Input: part model. Units: mm. Frame: model coordinates. Give positions to 0.01 mm unless a question says otherwise; leave off trailing zeros. Write each loop counter-clockwise with the first axis right and the second up, starting at its lowest first coordinate (ties: lowest second). Pieces come first, ordered by that corner, then holes.
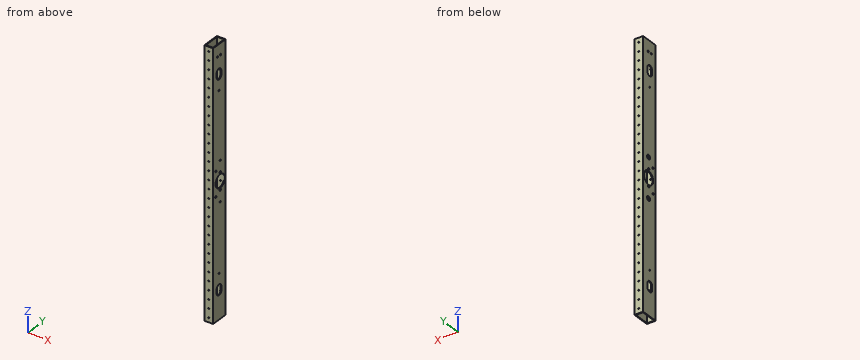
```python
from build123d import *

# Parameters (mm, degrees)
SKETCH1_W           = 25.4
SKETCH1_H           = 50.8
SKETCH1_W_2         = 20.32
SKETCH1_H_2         = 45.72
EXTRUDE_THIN1_DEPTH = 381
SKETCH3_R           = 1.5875
CUT_EXTRUDE2_DEPTH  = 51.8
LPATTERN1_COUNT     = 220
LPATTERN1_PITCH     = 25.4
SKETCH6_R           = 19.05
SKETCH6_R_2         = 3.175
CUT_EXTRUDE5_DEPTH  = 26.4
SKETCH4_R           = 9.525
CUT_EXTRUDE3_DEPTH  = 26.4
CUT_EXTRUDE6_START  = -22.86
SKETCH7_R           = 6.35
CUT_EXTRUDE6_DEPTH  = 2.54
SKETCH8_R           = 2.5273
CUT_EXTRUDE7_DEPTH  = 26.4
SKETCH9_R           = 2.0193
CUT_EXTRUDE8_DEPTH  = 26.4
SKETCH10_R          = 2.4892
CUT_EXTRUDE9_DEPTH  = 26.4
SKETCH11_R          = 2.413
CUT_EXTRUDE10_DEPTH = 26.4


with BuildPart() as part:
    # Sketch1 → Extrude-Thin1 (new body, symmetric)
    with BuildSketch(Plane.XY):
        with Locations((12.7, 25.4)):
            Rectangle(SKETCH1_W, SKETCH1_H)
        with Locations((12.7, 25.4)):
            Rectangle(SKETCH1_W_2, SKETCH1_H_2, mode=Mode.SUBTRACT)
    extrude(amount=EXTRUDE_THIN1_DEPTH, both=True)

    # Sketch3 → Cut-Extrude2 (cut, through all)
    with BuildSketch(Plane(origin=(0, 50.8, 0), x_dir=(1, 0, 0), z_dir=(0, 1, 0))):
        with Locations((12.7, -368.3)):
            Circle(SKETCH3_R)
    cut_extrude2 = extrude(amount=-CUT_EXTRUDE2_DEPTH, mode=Mode.SUBTRACT)

    # LPattern1: Cut-Extrude2 ×220
    with Locations(*[(0, 0, -i * LPATTERN1_PITCH) for i in range(1, LPATTERN1_COUNT)]):
        add(cut_extrude2, mode=Mode.SUBTRACT)

    # Sketch6 → Cut-Extrude5 (cut, through all)
    with BuildSketch(Plane(origin=(25.4, 0, 0), x_dir=(0, 0, -1), z_dir=(1, 0, 0))):
        with Locations((0, 28.7655)):
            Circle(SKETCH6_R)
        with Locations((23.8125, 28.7655)):
            Circle(SKETCH6_R_2)
        with Locations((-23.8125, 28.7655)):
            Circle(SKETCH6_R_2)
    extrude(amount=-CUT_EXTRUDE5_DEPTH, mode=Mode.SUBTRACT)

    # Sketch4 → Cut-Extrude3 (cut, through all)
    with BuildSketch(Plane(origin=(25.4, 0, 0), x_dir=(0, 0, -1), z_dir=(1, 0, 0))):
        with Locations((295.234514267, 23.876)):
            Circle(SKETCH4_R)
        with BuildLine():
            Line((304.124514267, 33.401), (295.234514267, 33.401))
            ThreePointArc((295.234514267, 33.401), (301.969706358, 30.611192091), (304.759514267, 23.876))
            ThreePointArc((304.759514267, 23.876), (301.969706356, 17.140807907), (295.234514261, 14.351))
            Line((295.234514261, 14.351), (304.124514267, 14.351))
            ThreePointArc((304.124514267, 14.351), (313.649514267, 23.876), (304.124514267, 33.401))
        make_face()
        with BuildLine():
            Line((295.234514267, 33.401), (292.694514267, 33.401))
            ThreePointArc((292.694514267, 33.401), (283.169514267, 23.876), (292.694514267, 14.351))
            Line((292.694514267, 14.351), (295.234514261, 14.351))
            ThreePointArc((295.234514261, 14.351), (285.709514267, 23.876000003), (295.234514267, 33.401))
        make_face()
    cut_extrude3 = extrude(amount=-CUT_EXTRUDE3_DEPTH, mode=Mode.SUBTRACT)

    # Mirror1: Cut-Extrude3 across plane
    add(cut_extrude3.mirror(Plane.XY), mode=Mode.SUBTRACT)

    # Sketch7 → Cut-Extrude6 (cut)
    with BuildSketch(Plane(origin=(25.4, 0, 0), x_dir=(0, 0, -1), z_dir=(1, 0, 0)).offset(CUT_EXTRUDE6_START)):
        with Locations((57.15, 28.7655)):
            Circle(SKETCH7_R)
        with Locations((-57.15, 28.7655)):
            Circle(SKETCH7_R)
    extrude(amount=-CUT_EXTRUDE6_DEPTH, mode=Mode.SUBTRACT)

    # Sketch8 → Cut-Extrude7 (cut, through all)
    with BuildSketch(Plane(origin=(25.4, 0, 0), x_dir=(0, 0, -1), z_dir=(1, 0, 0))):
        with Locations((-35.41150672, 10.9347)):
            Circle(SKETCH8_R)
        with Locations((35.41150672, 10.9347)):
            Circle(SKETCH8_R)
    extrude(amount=-CUT_EXTRUDE7_DEPTH, mode=Mode.SUBTRACT)

    # Sketch9 → Cut-Extrude8 (cut, through all)
    with BuildSketch(Plane.ZY):
        with Locations((252.689514267, 23.876)):
            Circle(SKETCH9_R)
    cut_extrude8 = extrude(amount=-CUT_EXTRUDE8_DEPTH, mode=Mode.SUBTRACT)

    # Mirror2: Cut-Extrude8 across plane
    add(cut_extrude8.mirror(Plane.XY), mode=Mode.SUBTRACT)

    # Sketch10 → Cut-Extrude9 (cut, through all)
    with BuildSketch(Plane.ZY):
        with Locations((348.574514267, 30.226)):
            Circle(SKETCH10_R)
        with Locations((348.574514267, 17.526)):
            Circle(SKETCH10_R)
    extrude(amount=-CUT_EXTRUDE9_DEPTH, mode=Mode.SUBTRACT)

    # Sketch11 → Cut-Extrude10 (cut, through all)
    with BuildSketch(Plane.ZY):
        with Locations((-57.15, 28.7655)):
            Circle(SKETCH11_R)
        with Locations((57.15, 28.7655)):
            Circle(SKETCH11_R)
    extrude(amount=-CUT_EXTRUDE10_DEPTH, mode=Mode.SUBTRACT)


solid = part.part
```
Q1. Section B-B, the plane z = -76. Return the cut outline in (x, y), then the cut area to 3 significant figures.
Q2. Pin query (flat end, axial travel): pin 1 (2.5 mm diameter, centred on x = 12.7, z = 266.7, fed in from -Y). Return the tip coordinate at first contact, or that it passes through.
Q3. Section A-A, the plane x = 7. Return the cut outline in (y, z).
Q4. Material intervals for line 1 along Y through (x, z) = (13, -262); line 2 along X through (y, z) = (28, -161.5); line 3 along Z through (x, y) = (23, 19), sorted ascending.
Solutions:
1. outline: (0, 0) - (25.4, 0) - (25.4, 50.8) - (0, 50.8) - close; hole (2.54, 2.54) - (22.86, 2.54) - (22.86, 48.26) - (2.54, 48.26) - close
1. area: 361 mm2
2. pin 1: passes through
3. outline: (0, -381) - (2.54, -381) - (2.54, 381) - (0, 381) - close; (48.26, -381) - (50.8, -381) - (50.8, 381) - (48.26, 381) - close
4. line 1: y = 0 to 2.54, 48.26 to 50.8
4. line 2: x = 0 to 2.54, 22.86 to 25.4
4. line 3: z = -381 to -312.31, -284.51 to -16.36, 16.36 to 284.51, 312.31 to 346.57, 350.58 to 381
